Geometry: final body of the model. Coordinates: model frame, mm. Face numbers are marked on the shaded views. A direction names the side the tool comes from. Give positions to 0.01 mm unless a question says otherwise; leave off trailing zeros. Loops run counter-clockwise (first coordinate to the right, second up) from the corner with the lowest first, then second, coordinate; pieces in that order, holes last.
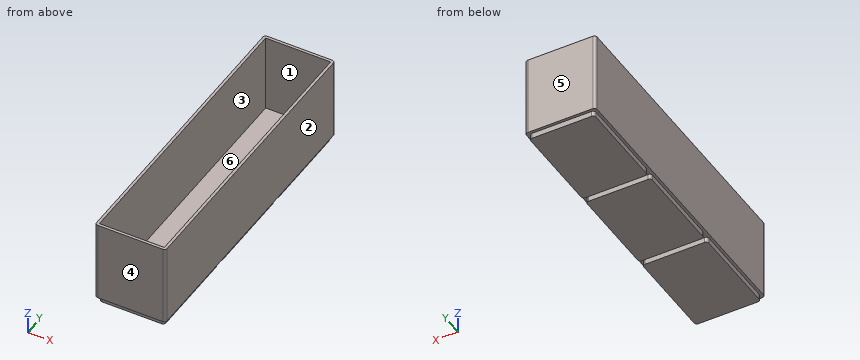
from build123d import *

# Parameters (mm, degrees)
F0_W     = 35
F0_H     = 50
F1_DEPTH = 3
F0_H_2   = 1.5
F2_DEPTH = 1.5
F3_DEPTH = 44
F4_R     = 1.5


with BuildPart() as f1:
    # F0 (on Top) → F1 (new body)
    with BuildSketch(Plane.XY):
        with Locations((19, 132.5)):
            Rectangle(F0_W, F0_H)
        with Locations((19, 79.5)):
            Rectangle(F0_W, F0_H)
        with Locations((19, 26.5)):
            Rectangle(F0_W, F0_H)
    extrude(amount=-F1_DEPTH)

    # F0 (on Top) → F2 (join)
    with BuildSketch(Plane.XY):
        Polygon((0, 159), (0, 106), (1.5, 106), (1.5, 107.5), (1.5, 157.5), (36.5, 157.5), (36.5, 107.5), (36.5, 106), (38, 106), (38, 159), align=None)
        with Locations((19, 132.5)):
            Rectangle(F0_W, F0_H)
        with Locations((19, 105.25)):
            Rectangle(F0_W, F0_H_2)
        with Locations((19, 106.75)):
            Rectangle(F0_W, F0_H_2)
        Polygon((36.5, 53), (38, 53), (38, 106), (36.5, 106), (36.5, 104.5), (36.5, 54.5), align=None)
        Polygon((0, 106), (0, 53), (1.5, 53), (1.5, 54.5), (1.5, 104.5), (1.5, 106), align=None)
        with Locations((19, 79.5)):
            Rectangle(F0_W, F0_H)
        with Locations((19, 53.75)):
            Rectangle(F0_W, F0_H_2)
        with Locations((19, 52.25)):
            Rectangle(F0_W, F0_H_2)
        with Locations((19, 26.5)):
            Rectangle(F0_W, F0_H)
        Polygon((0, 53), (0, 0), (38, 0), (38, 53), (36.5, 53), (36.5, 51.5), (36.5, 1.5), (1.5, 1.5), (1.5, 51.5), (1.5, 53), align=None)
    extrude(amount=F2_DEPTH)

    # F0 (on Top) → F3 (join)
    with BuildSketch(Plane.XY):
        Polygon((0, 159), (0, 106), (1.5, 106), (1.5, 107.5), (1.5, 157.5), (36.5, 157.5), (36.5, 107.5), (36.5, 106), (38, 106), (38, 159), align=None)
        Polygon((0, 106), (0, 53), (1.5, 53), (1.5, 54.5), (1.5, 104.5), (1.5, 106), align=None)
        Polygon((36.5, 53), (38, 53), (38, 106), (36.5, 106), (36.5, 104.5), (36.5, 54.5), align=None)
        Polygon((0, 53), (0, 0), (38, 0), (38, 53), (36.5, 53), (36.5, 51.5), (36.5, 1.5), (1.5, 1.5), (1.5, 51.5), (1.5, 53), align=None)
    extrude(amount=F3_DEPTH)

    # F4
    f4_edges = [f1.edges().sort_by_distance(p)[0] for p in [
        (0, 159, 22),
        (38, 159, 22),
        (36.5, 157.5, -1.5),
        (1.5, 157.5, -1.5),
        (36.5, 107.5, -1.5),
        (1.5, 107.5, -1.5),
        (1.5, 104.5, -1.5),
        (36.5, 104.5, -1.5),
        (36.5, 54.5, -1.5),
        (36.5, 51.5, -1.5),
        (1.5, 51.5, -1.5),
        (1.5, 54.5, -1.5),
        (36.5, 1.5, -1.5),
        (38, 0, 22),
        (1.5, 1.5, -1.5),
        (0, 0, 22),
    ]]
    fillet(f4_edges, radius=F4_R)


solid = f1.part
Item 1: Section query B-B on x = 12. Return loops of the section in (y, z), plus the area to 3 significant figures.
Values follow:
outline: (0, 0) - (1.5, 0) - (1.5, -3) - (51.5, -3) - (51.5, 0) - (54.5, 0) - (54.5, -3) - (104.5, -3) - (104.5, 0) - (107.5, 0) - (107.5, -3) - (157.5, -3) - (157.5, 0) - (159, 0) - (159, 44) - (157.5, 44) - (157.5, 1.5) - (1.5, 1.5) - (1.5, 44) - (0, 44) - close
area: 816 mm2
Item 2: Pin query (flat end, axial travel): pin 1 (2.5 mm diameter, centred on x = 24.5, z = -2, fed in from +Y); pin 2 (0.9 mm diameter, centred on x = 20, z = -1, fed in from -Y); pin 3 (3.5 mm diameter, centred on x = 17.5, z = -1.5, fed in from -Y); pin 4 (0.9 mm diameter, centred on y = 131, z = -2, fed in from -X). Return the tip coordinate at first contact, or that it passes through.
Values follow:
pin 1: stops at y = 157.5
pin 2: stops at y = 1.5
pin 3: stops at y = 0
pin 4: stops at x = 1.5
Item 3: Set-up query: the marked faces 5 and 6. Return all of +Z, -Z, +X, -X, +Y, -Y with unobstructed straight access to the full face (end or side cutting, diameter ignored); none if empty.
Values follow:
face 5: +Z, -Z, +X, -X, +Y
face 6: +Z
Item 4: Ray query, probe 1 along X at (y, z) = (49, 7); probe 2 along Y at (x, z) = (25, 38); probe 3 along Z at (x, y) = (4, 18). Return the intervals inside material, ascending.
Values follow:
probe 1: x = 0 to 1.5, 36.5 to 38
probe 2: y = 0 to 1.5, 157.5 to 159
probe 3: z = -3 to 1.5
Item 5: Draft query along X for the marked faces 1, 2, 3 and 4. Return one class per face: +X half, -X half, draft (parallel to the pull), parting line (faces both ways), or undercut.
Values follow:
face 1: undercut
face 2: +X half
face 3: undercut
face 4: draft
Item 6: Section query C-C on y = 143. Return loops of the section in (x, z), plus the area to 4 significant figures.
Values follow:
outline: (0, 0) - (1.5, 0) - (1.5, -3) - (36.5, -3) - (36.5, 0) - (38, 0) - (38, 44) - (36.5, 44) - (36.5, 1.5) - (1.5, 1.5) - (1.5, 44) - (0, 44) - close
area: 289.5 mm2
Item 7: Section query A-A on z = 30.5. Return loops of the section in (x, y), plus the area to 3 significant figures.
Values follow:
outline: (0, 1.5) arc R1.5 ccw to (1.5, 0) - (36.5, 0) arc R1.5 ccw to (38, 1.5) - (38, 157.5) arc R1.5 ccw to (36.5, 159) - (1.5, 159) arc R1.5 ccw to (0, 157.5) - close; hole (1.5, 1.5) - (36.5, 1.5) - (36.5, 157.5) - (1.5, 157.5) - close
area: 580 mm2
